Answer from the drawing. Dimensions are ordinates in mm from the lowest x, y and z of the part. A direction names the side the tool comes from. Give positions to 0.01 mm unless a question says otherwise; leave off trailing zeros. Order: outer loops, then holes, each group sorted by start corner. A loop starts at its lowest first (then second) coordinate and runs counter-clockwise, first axis right, second up. Notation, with made-up numbers: (9.5, -6.75) - (15.5, -6.75) arc R34 cw to (15.5, 25.25) - close; hole circle Ø9 at (7.5, -16). An arc over 180 degrees is marked (long way). Answer in a Markdown table with one row per item.
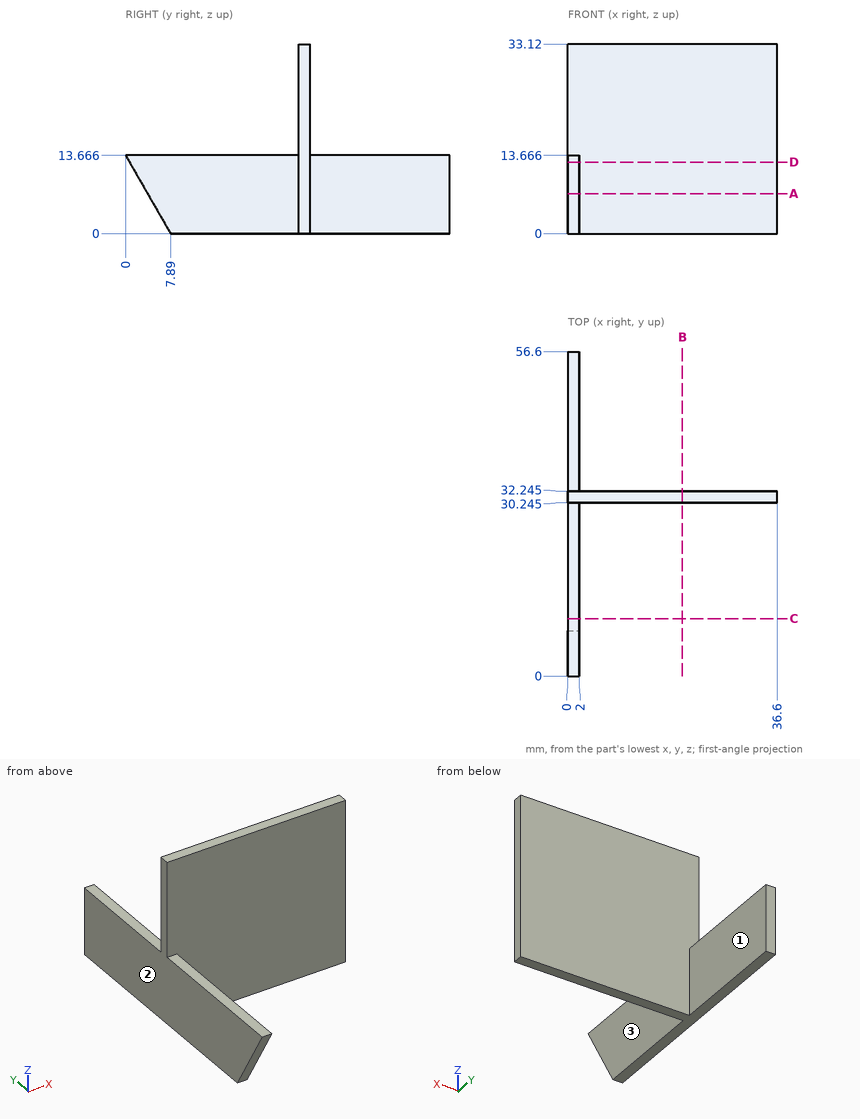
Item 1: Find section B-B on x = 20. Write down the section's boundary in (y, z) (3 decimals).
Answer block:
| item | result |
|---|---|
| outline | (30.245, 0) - (32.245, 0) - (32.245, 33.12) - (30.245, 33.12) - close |
Item 2: Consider line 1 (Y direction, x = 24, z = 17) (3 decimals); line 2 (X direction, y = 25, z = 7). Determine where each line is inside the solid, lowest interval first.
Answer block:
| item | result |
|---|---|
| line 1 | 30.245 to 32.245 |
| line 2 | 0 to 2 |
Item 3: Find section A-A on z = 7. Write down the section's boundary in (x, y) (1 decimal).
Answer block:
| item | result |
|---|---|
| outline | (0, 3.8) - (2, 3.8) - (2, 30.2) - (36.6, 30.2) - (36.6, 32.2) - (2, 32.2) - (2, 56.6) - (0, 56.6) - close |
Item 4: Which of the six approach directions +Z, -Z, +X, -X, +Y, -Y give full straight-line access (tool end or side, diameter ignored) to the marked faces 1, 2 and 3?
Answer block:
| item | result |
|---|---|
| face 1 | +Z, -Z, +X, +Y |
| face 2 | +Z, -Z, -X, +Y, -Y |
| face 3 | +Z, -Z, +X, -Y |
Item 5: Find section C-C on y = 10. Write down the section's boundary in (x, z), then the cut area to 3 significant figures.
Answer block:
| item | result |
|---|---|
| outline | (0, 0) - (2, 0) - (2, 13.67) - (0, 13.67) - close |
| area | 27.3 mm² |
Item 6: Find section D-D on z = 12.5. Write down the section's boundary in (x, y) (3 decimals), then the cut area to 3 significant figures.
Answer block:
| item | result |
|---|---|
| outline | (0, 0.673) - (2, 0.673) - (2, 30.245) - (36.6, 30.245) - (36.6, 32.245) - (2, 32.245) - (2, 56.6) - (0, 56.6) - close |
| area | 181 mm² |
Item 7: Each of these flat-tipped pins is pushed along its axis until it touches: P1, Ø16.5, axis at x = 14.5, z = 17, coming from the +Y side (3 decimals); P2, Ø2, axis at x = 9.5, z = 7.5, coming from the -Y side (3 decimals); P3, Ø4, axis at y = 20.5, z = 5, coming from the +X side. Where does it stop, or does it pass through?
Answer block:
| item | result |
|---|---|
| P1 | y = 32.245 |
| P2 | y = 30.245 |
| P3 | x = 2 |
